Build history of the part. All positions in model axes, mm. Round coordinates to 2 decimals unless told otherwise and drop trailing zeros. Loops run counter-clockwise (first coordinate to the right, second up) from the corner with the lowest first, then second, coordinate; pieces in that order, holes last. Notation, with made-up numbers: (79, -24.5) - (117, -24.5) arc R13 ccw to (117, -0.5) - close; hole circle Ø3 at (-35, -2.75). An arc over 180 degrees is marked (long way). Answer as CSV lines item,"result". Start each with the question number.
```python
from build123d import *

# Parameters (mm, degrees)
F1_DEPTH = 85.725
F3_DEPTH = 50.8
F4_R     = 1.5875
F5_DEPTH = 127


with BuildPart() as f1:
    # F0 (on Front) → F1 (new body)
    with BuildSketch(Plane.XZ):
        Polygon((-67.6071290719, 80.2582807616), (-118.4071290719, 80.2582807616), (55.9836195711, -100.0221879884), (106.7836195711, -100.0221879884), align=None)
    extrude(amount=F1_DEPTH)

    # F2 (on face) → F3 (cut)
    with BuildSketch(Plane(origin=(5.1810656307, 0, 5.0118014468), x_dir=(0, 1, 0), z_dir=(0.71875, 0, 0.6952686082))):
        with BuildLine():
            Line((-58.7375, -3.2592461708), (-26.9875, -3.2592461708))
            ThreePointArc((-26.9875, -3.2592461708), (-42.8625, 12.6157538292), (-58.7375, -3.2592461708))
        make_face()
        with BuildLine():
            ThreePointArc((-58.7375, -3.2592461708), (-42.8625, -19.1342461708), (-26.9875, -3.2592461708))
            Line((-26.9875, -3.2592461708), (-58.7375, -3.2592461708))
        make_face()
    extrude(amount=-F3_DEPTH, mode=Mode.SUBTRACT)

    # F4 (on face) → F5 (cut)
    with BuildSketch(Plane(origin=(0, 0, 0), x_dir=(-1, 0, 0), z_dir=(0, 1, 0))):
        with Locations((-44.76928715, -62.1007793102)):
            Circle(F4_R)
        with Locations((57.455530428, 43.4951331483)):
            Circle(F4_R)
    extrude(amount=-F5_DEPTH, mode=Mode.SUBTRACT)


solid = f1.part
```
Q1. Pin check, flat tips, straight feed: pin 1 Ø6 at (y, z) = (-19, -30.5) entering from +X; pin 2 Ø5 at (y, z) = (-18, -71) entering from +X; pin 3 Ø6 at (x, y) = (69.5, -72) entering from +Z. Stop position of each tip, or through.
Q2. Band-saw the part on A-A, the plane y = -46. List the corners of the cut face in (x, z) (1 decimal), then the cut area to 3 significant figures.
Q3. Band-saw the part on D-D, the plane y = -7. List the corners of the cut face in (x, z) (1 decimal), then the cut area to 3 significant figures.
Q4. Band-saw the part on C-C, the plane x = -90. List the corners of the cut face in (y, z) (3 decimals).
Q5. Two-plate mould, pull along Z, no slides. Class faces 1 (the cylindrical face through (-5, -27, -10.3)), 2 (the flat face through (-32.43, -42.26, -8.62)), 3 (the flat face through (-6, -85.725, -9)): released by +Z, released by -Z, zero draft, split by the parting line, or undercut.
Q6. Band-saw the part on B-B, the plane y = -34. List the corners of the cut face in (x, z) (1 decimal).
Q7. Wall check: probe 1 along Z at (x, y) = (-82.5, -44); probe 2 along X at (y, z) = (-28, -32.5); probe 3 along X at (y, z) = (-20, -71). Give the ranges that are in metal, low to high. Write a range as [from, to].
Reported:
1,pin 1,"stops at x = 42.43"
1,pin 2,"stops at x = 81.13"
1,pin 3,"stops at z = -58.38"
2,outline,"(-118.4, 80.3) - (-29.6, -11.5) - (-3.4, 13.9) - (-67.6, 80.3) - close; (-8, -33.9) - (56, -100) - (106.8, -100) - (18.3, -8.5) - close; hole circle Ø3.2 at (-57.5, 43.5); hole circle Ø3.2 at (44.8, -62.1)"
2,area,"8,010 mm2"
3,outline,"(-118.4, 80.3) - (56, -100) - (106.8, -100) - (-67.6, 80.3) - close; hole circle Ø3.2 at (-57.5, 43.5); hole circle Ø3.2 at (44.8, -62.1)"
3,area,"9,140 mm2"
4,outline,"(-85.725, 50.892) - (0, 50.892) - (0, 80.258) - (-85.725, 80.258) - close"
5,face 1,"undercut"
5,face 2,"released by -Z"
5,face 3,"zero draft"
6,outline,"(-118.4, 80.3) - (-28, -13.3) - (-1.7, 12.1) - (-67.6, 80.3) - close; (-9.6, -32.2) - (56, -100) - (106.8, -100) - (16.6, -6.8) - close; hole circle Ø3.2 at (-57.5, 43.5); hole circle Ø3.2 at (44.8, -62.1)"
7,probe 1,"z = [43.14, 80.26]"
7,probe 2,"x = [-9.33, 41.47]"
7,probe 3,"x = [27.91, 78.71]"
